Verification items for this drawing (mm, ordinates from the low corner). Round coordinates to 2 decimals unless told otherwise and drop trailing zeros. Order: outer loops, then holes, each group sorted by start corner. A loop starts at its lowest first (then second) coordinate and runs counter-clockwise, first axis right, second up. Notation, with made-up numbers: (20.25, 68) - (55.25, 68) arc R16 ccw to (55.25, 81) - close; hole circle Ø1 at (73.25, -4). An arc over 180 degrees is marked (long way). Return JSON: item names as keys, results as strings. Group by question number.
Q1. Material ranges on line 1 along Y through (x, z) = (167, 35.5); line 2 along Z through (x, y) = (174.5, 50), recorded low to high.
Q2. Gauge pin test, flat ends, axial feed: pin 1 Ø12.5 at (y, z) = (41, 29) entering from -X; pin 2 Ø2 at (x, y) = (194, 43.5) entering from +Z. Record the tip position at first contact, or that the pin passes through.
Q3. Sectioned sample at B-B, the plane x = 443. Record the cut outline in (y, z), then the cut area to 3 significant figures.
Q4. Sectioned sample at A-A, the plane y = 45.5. Record the cut outline in (x, z).
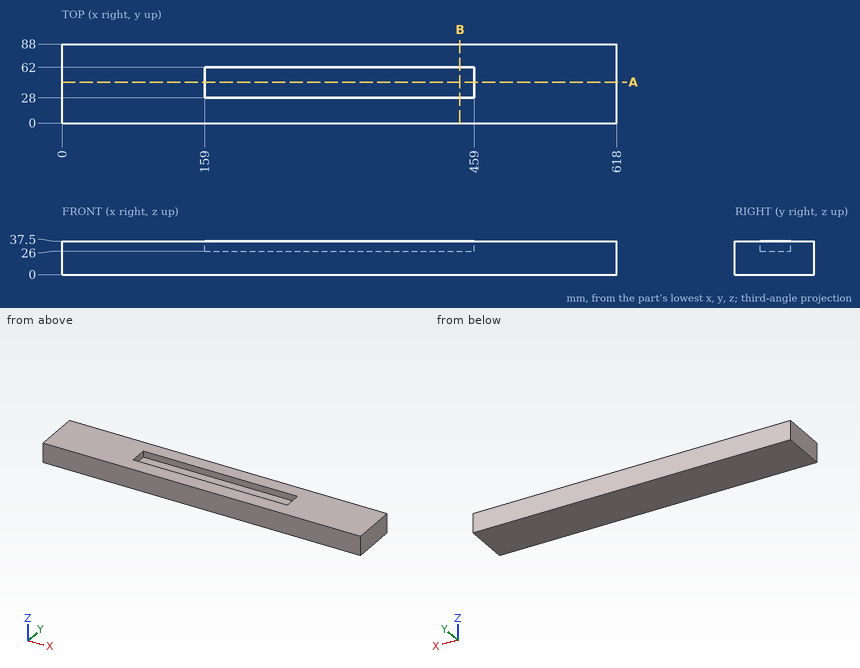
Reply:
{
 "1": {"line 1": "0 to 28, 62 to 88", "line 2": "0 to 26"},
 "2": {"pin 1": "x = 0", "pin 2": "z = 26"},
 "3": {"outline": "(0, 0) - (88, 0) - (88, 37.5) - (62, 37.5) - (62, 26) - (28, 26) - (28, 37.5) - (0, 37.5) - close", "area": "2,910 mm^2"},
 "4": {"outline": "(0, 0) - (618, 0) - (618, 37.5) - (459, 37.5) - (459, 26) - (159, 26) - (159, 37.5) - (0, 37.5) - close"}
}
